Part model, mm, in its own coordinate system. Face numbers are marked on the shaded views. A direction names the side the tool comes from. Round coordinates to 2 decimals unless told otherwise and drop trailing zeros. Loops run counter-clockwise (first coordinate to the right, second up) from the corner with the lowest first, then second, coordinate; pieces in that order, holes last. Notation, with made-up numbers: M 27,82 L 63,82 A16 ccw 63,113 Z; hole C 89.5,55 d10. An arc over 180 degrees is marked long. Answer as CSV lines item,"result". Start each with the question number.
Item 1: Band-saw the part on A-A (x = -203). Give the cut face in (y, z).
Item 2: Wall check: line 1 (Y direction, x = -203, z = 88.7); line 2 (X direction, y = 21.25, z = 92.5); line 3 (Z direction, x = -197.5, y = 29.5). Give the ranges that are in metal, low to high.
Item 3: Band-saw the part on D-D (x = -197). Give the cut face in (y, z).
Item 4: Band-saw the part on C-C (y = 21.75). Give the cut face in (x, z), and give its area (3 significant figures).
Item 5: Band-saw the part on B-B (z = 91.5). Give the cut face in (x, y), and give its area (3 significant figures).
Item 6: Drop flat-ended pins along their axis: pin 1 Ø2 at (y, z) = (38.5, 94.5) entering from -X; pin 2 Ø1 at (x, y) = (-204.5, 23) entering from +Z; pin 3 Ø0.6 at (x, z) = (-194, 93.5) entering from -Y; pin 4 Ø2.5 at (x, y) = (-203, 40) entering from -Z. Give the stop position or say it passes through.
Item 7: Mould opens along Y. For the marked faces 1, 2 and 3 say: pulls with the +Y half, pulls with the -Y half, needs draft (parallel to the pull), parting line crosses it, or undercut.
Item 8: Which spindle directions (+Z, -Z, +X, -X, +Y, -Y) get a long thin tool onto all of the face, cutting with end or side? Do the marked faces 4, 5, 6 and 7. Say none if no direction does.
```python
from build123d import *

# Parameters (mm, degrees)
MAIN_PROFILE_SKETCH_W     = 22
MAIN_PROFILE_SKETCH_H     = 28
MAIN_PROFILE_SKETCH_R     = 1.7
MAIN_EXTRUSION_DEPTH      = 2
DETAIL_PROFILE_2_SKETCH_W = 2
DETAIL_PROFILE_2_SKETCH_H = 22
DETAIL_EXTRUSION_2_DEPTH  = 6


with BuildPart() as part:
    # Main Profile Sketch → Main Extrusion (new body)
    with BuildSketch(Plane.XY.offset(88)):
        with Locations((-203, 29)):
            Rectangle(MAIN_PROFILE_SKETCH_W, MAIN_PROFILE_SKETCH_H)
        with Locations((-203, 18)):
            Circle(MAIN_PROFILE_SKETCH_R, mode=Mode.SUBTRACT)
        with Locations((-203, 40)):
            Circle(MAIN_PROFILE_SKETCH_R, mode=Mode.SUBTRACT)
    extrude(amount=MAIN_EXTRUSION_DEPTH)

    # Detail Profile 2 Sketch → Detail Extrusion 2 (add)
    with BuildSketch(Plane.XY.offset(90)):
        with Locations((-194, 29)):
            Rectangle(DETAIL_PROFILE_2_SKETCH_W, DETAIL_PROFILE_2_SKETCH_H)
        with Locations((-212, 29)):
            Rectangle(DETAIL_PROFILE_2_SKETCH_W, DETAIL_PROFILE_2_SKETCH_H)
    extrude(amount=DETAIL_EXTRUSION_2_DEPTH)


solid = part.part
```
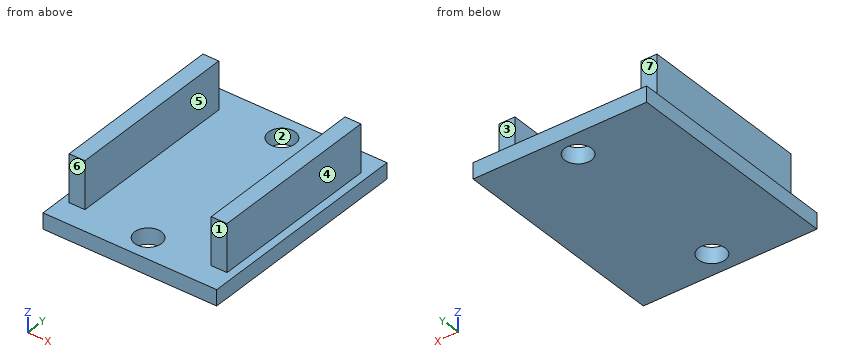
Answer block:
1,outline,"M 15,88 L 16.3,88 L 16.3,90 L 15,90 Z; M 19.7,88 L 38.3,88 L 38.3,90 L 19.7,90 Z; M 41.7,88 L 43,88 L 43,90 L 41.7,90 Z"
2,line 1,"y = 15 to 16.3, 19.7 to 38.3, 41.7 to 43"
2,line 2,"x = -213 to -211, -195 to -193"
2,line 3,"z = 88 to 90"
3,outline,"M 15,88 L 43,88 L 43,90 L 15,90 Z"
4,outline,"M -214,88 L -192,88 L -192,90 L -193,90 L -193,96 L -195,96 L -195,90 L -211,90 L -211,96 L -213,96 L -213,90 L -214,90 Z"
4,area,"68.0 mm^2"
5,outline,"M -213,18 L -211,18 L -211,40 L -213,40 Z; M -195,18 L -193,18 L -193,40 L -195,40 Z"
5,area,"88.0 mm^2"
6,pin 1,"stops at x = -213"
6,pin 2,"stops at z = 90"
6,pin 3,"stops at y = 18"
6,pin 4,"passes through"
7,face 1,"pulls with the -Y half"
7,face 2,"undercut"
7,face 3,"pulls with the +Y half"
8,face 4,"+Z, +X, +Y, -Y"
8,face 5,"+Z, +Y, -Y"
8,face 6,"+Z, +X, -X, -Y"
8,face 7,"+Z, +X, -X, +Y"
